For this review, take the finished solid that the model builds, in its own axes (mm). Face numbers are marked on the shaded views. A direction names the side the tool comes from. Round coordinates to 2 decimals unless told otherwise and drop trailing zeros. Order: outer loops, then holes, each group sorted by start corner. A loop starts at its lowest first (then second) coordinate and runs counter-clockwise, first axis right, second up. Notation, with made-up numbers: (87.5, 82) - (108.5, 82) arc R20 cw to (108.5, 95) - close; hole circle Ø4 at (-24, 68.5). An arc over 180 degrees is marked (long way). One line per item, written item: value.
```python
from build123d import *

# Parameters (mm, degrees)
SKETCH_1_W          = 100
SKETCH_1_H          = 150
EXTRUDE_1_DEPTH     = 20
SKETCH_2_R          = 15
CUT_EXTRUDE_1_DEPTH = 20
SKETCH_3_W          = 25
SKETCH_3_H          = 30
CUT_EXTRUDE_2_DEPTH = 20
SKETCH_4_W          = 15
SKETCH_4_H          = 90
EXTRUDE_2_DEPTH     = 60
SKETCH_6_W          = 15
SKETCH_6_H          = 90
EXTRUDE_3_DEPTH     = 60
CUT_EXTRUDE_3_REACH = 140.654
CUT_EXTRUDE_4_REACH = 112.68
SKETCH_9_W          = 25
SKETCH_9_H          = 25
SKETCH_10_W         = 20
SKETCH_10_H         = 10
CUT_EXTRUDE_5_DEPTH = 139.654246239


with BuildPart() as part:
    # Эскиз1 → Бобышка-Вытянуть1 (new body)
    with BuildSketch(Plane(origin=(0, 0, 0), x_dir=(1, 0, 0), z_dir=(0, 1, 0))):
        Rectangle(SKETCH_1_W, SKETCH_1_H)
    extrude(amount=-EXTRUDE_1_DEPTH)

    # Эскиз2 → Вырез-Вытянуть1 (cut)
    with BuildSketch(Plane(origin=(0, 0, 0), x_dir=(1, 0, 0), z_dir=(0, 1, 0))):
        with Locations((-50, -45)):
            Circle(SKETCH_2_R)
    extrude(amount=-CUT_EXTRUDE_1_DEPTH, mode=Mode.SUBTRACT)

    # Эскиз3 → Вырез-Вытянуть2 (cut)
    with BuildSketch(Plane(origin=(0, 0, 0), x_dir=(1, 0, 0), z_dir=(0, 1, 0))):
        with Locations((22.5, -60)):
            Rectangle(SKETCH_3_W, SKETCH_3_H)
    extrude(amount=-CUT_EXTRUDE_2_DEPTH, mode=Mode.SUBTRACT)

    # Эскиз4 → Бобышка-Вытянуть2 (add)
    with BuildSketch(Plane(origin=(0, 0, 0), x_dir=(1, 0, 0), z_dir=(0, 1, 0))):
        with Locations((2.5, 0)):
            Rectangle(SKETCH_4_W, SKETCH_4_H)
    extrude(amount=EXTRUDE_2_DEPTH)

    # Эскиз6 → Бобышка-Вытянуть3 (add)
    with BuildSketch(Plane(origin=(0, 0, 0), x_dir=(1, 0, 0), z_dir=(0, 1, 0))):
        with Locations((42.5, 0)):
            Rectangle(SKETCH_6_W, SKETCH_6_H)
    extrude(amount=EXTRUDE_3_DEPTH)

    # Эскиз7 → Вырез-Вытянуть3 (cut, up to next)
    with BuildSketch(Plane(origin=(50, 0, 0), x_dir=(0, 0, -1), z_dir=(1, 0, 0)), mode=Mode.PRIVATE) as cut_extrude_3_sk1:
        with BuildLine():
            Line((-45, 40), (-45, 10))
            ThreePointArc((-45, 10), (-30, 25), (-45, 40))
        make_face()
    cut_extrude_3_tool1 = extrude(cut_extrude_3_sk1.sketch, amount=-CUT_EXTRUDE_3_REACH, mode=Mode.PRIVATE) & part.part
    add(cut_extrude_3_tool1.solids().sort_by_distance((50, 25, 38.633802))[0], mode=Mode.SUBTRACT)

    # Эскиз9 → Вырез-Вытянуть4 (cut, up to next)
    with BuildSketch(Plane.ZY.offset(5), mode=Mode.PRIVATE) as cut_extrude_4_sk1:
        with Locations((32.5, 22.5)):
            Rectangle(SKETCH_9_W, SKETCH_9_H)
    cut_extrude_4_tool1 = extrude(cut_extrude_4_sk1.sketch, amount=-CUT_EXTRUDE_4_REACH, mode=Mode.PRIVATE) & part.part
    add(cut_extrude_4_tool1.solids().sort_by_distance((-5, 22.5, 32.5))[0], mode=Mode.SUBTRACT)

    # Эскиз10 → Вырез-Вытянуть5 (cut, through all)
    with BuildSketch(Plane(origin=(50, 0, 0), x_dir=(0, 0, -1), z_dir=(1, 0, 0))):
        with Locations((65, -15)):
            Rectangle(SKETCH_10_W, SKETCH_10_H)
    extrude(amount=-CUT_EXTRUDE_5_DEPTH, mode=Mode.SUBTRACT)


solid = part.part
```
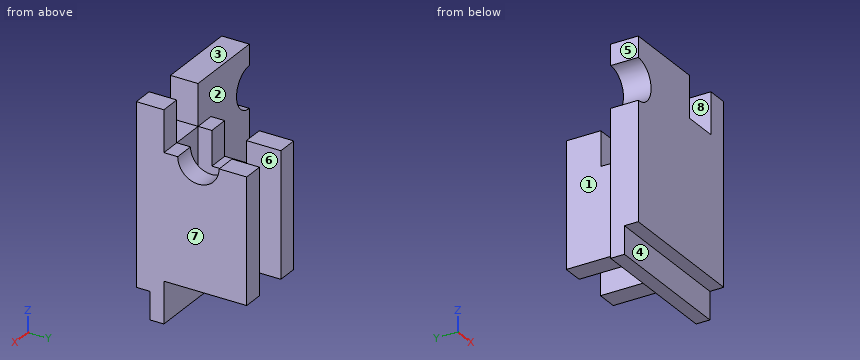
Item 1: Wall thickness on line 1 (X direction, y = 5.5, z = 4); line 2 (Z direction, x = 7.5, y = 17); line 3 (Y direction, x = -19, z = -67): over which ranges is each line inside the solid? List them lowest first.
Returned:
line 1: -5 to 10, 35 to 50
line 2: -45 to 20
line 3: -10 to 0
Item 2: Take a section at C-C (z = -6.5). Write out the cut boundary in (x, y).
Returned:
outline: (-50, -20) - (50, -20) - (50, 60) - (35, 60) - (35, 0) - (10, 0) - (10, 60) - (-5, 60) - (-5, 0) - (-50, 0) - close
Item 3: Take a section at A-A (y = 25). Write out the cut boundary in (x, z), plus the area to 3 significant figures.
Returned:
outline: (-5, -45) - (10, -45) - (10, 20) - (-5, 20) - close; (35, -45) - (50, -45) - (50, 30) - (35, 30) - close
area: 2,100 mm^2
Item 4: For P1, Ø12, axis at x = -1, y = 23, coming from the +Z side; P2, Ø10, axis at x = -2.5, z = -67, coming from the -Y side; P3, Ø10, axis at x = 16, y = 42, coming from the +Z side; P4, Ø16.5, axis at x = 44.5, y = 52, coming from the +Z side, all flat-tipped, find the tip position at first contact; note any pin that passes through.
Returned:
P1: z = 20
P2: y = -10
P3: through
P4: z = 45
Item 5: The part is to be moulded in two halves that separate along X. For the marked faces 1, 2 and 3, say which applies: +X half, -X half, draft (parallel to the pull), parting line (faces both ways), or undercut.
Returned:
face 1: -X half
face 2: undercut
face 3: draft
Item 6: Take a section at B-B (z = 42.5). Write out the cut boundary in (x, y), plus the area to 3 significant figures.
Returned:
outline: (-35.21, -20) - (50, -20) - (50, 10.21) - (35, 10.21) - (35, 0) - (10, 0) - (10, 10) - (-5, 10) - (-5, 0) - (-35.21, 0) - close; (-5, 35) - (10, 35) - (10, 60) - (-5, 60) - close; (35, 39.79) - (50, 39.79) - (50, 60) - (35, 60) - close
area: 2,690 mm^2
Item 7: Machinability: for the marked faces 4, 5, 6, 7 and 8, which of the approach directions +Z, -Z, +X, -X, +Y, -Y give a long, thin tool a straight path to every point of the face, cutting with its end or side? Answer none if there is none.
Returned:
face 4: -Z, +X, -X, -Y
face 5: +Z, -Z, -X, +Y, -Y
face 6: +Z, -Z, +Y
face 7: +Z, -Z, +X, +Y, -Y
face 8: +Z, +Y, -Y
Item 8: Take a section at D-D (y = -4). Write out the cut boundary in (x, z), plus the area to 3 significant figures.
Returned:
outline: (-50, -75) - (50, -75) - (50, 75) - (35, 75) - (35, 45) - (10, 45) - (10, 75) - (-50, 75) - (-50, 60) arc R15 cw to (-50, 30) - close
area: 13,900 mm^2
